from build123d import *
from build123d.topology import SkipClean

# Parameters (mm, degrees)
EXTRUDE_1_DEPTH        = 4
EXTRUDE_3_DEPTH        = 6
CHAMFER_1_SIZE         = 3
SKETCH_5_R             = 0.85
CUT_EXTRUDE_1_DEPTH    = 4
PATTERN_LINEAR_1_COUNT = 4
PATTERN_LINEAR_1_PITCH = 8
CUT_EXTRUDE_2_DEPTH    = 2.5
CUT_EXTRUDE_3_REACH    = 41.439
SKETCH_7_R             = 1.35
SKETCH_8_R             = 6
EXTRUDE_4_DEPTH        = 1.5
FILLET_1_R             = 0.5
SKETCH_9_R             = 5
CUT_EXTRUDE_4_DEPTH    = 3.6
SKETCH_10_R            = 3.55
CUT_EXTRUDE_5_DEPTH    = 3.6
CUT_EXTRUDE_6_DEPTH    = 0.8
CUT_EXTRUDE_7_DEPTH    = 40.958228189
FILLET_2_R             = 2
CHAMFER_2_SIZE         = 1
EXTRUDE_5_DEPTH        = 10


with BuildPart() as part:
    # ｽｹｯﾁ1 → ﾎﾞｽ - 押し出し1 (new body)
    with BuildSketch(Plane(origin=(0, 0, 0), x_dir=(1, 0, 0), z_dir=(0, 1, 0))):
        with BuildLine():
            Line((-7.9, 0), (-7.9, -38))
            Line((-7.9, -38), (7.9, -38))
            Line((7.9, -38), (7.9, 0))
            ThreePointArc((7.9, 0), (0, 7.9), (-7.9, 0))
        make_face()
    extrude(amount=EXTRUDE_1_DEPTH)

    # ｽｹｯﾁ4 → ﾎﾞｽ - 押し出し3 (add)
    with BuildSketch(Plane.XY.offset(38)):
        Polygon((-7, -5.5), (-4.5, -5.5), (-3, -2), (3, -2), (4.5, -5.5), (7, -5.5), (7.9, -2), (7.9, 0), (-7.9, 0), (-7.9, -2), align=None)
    extrude(amount=-EXTRUDE_3_DEPTH)

    # 面取り1
    chamfer_1_edges = [part.edges().sort_by_distance(p)[0] for p in [
        (0, 4, 38),
    ]]
    chamfer(chamfer_1_edges, length=CHAMFER_1_SIZE)

    # ｽｹｯﾁ5 → ｶｯﾄ - 押し出し1 (cut)
    with BuildSketch(Plane(origin=(0, 4, 0), x_dir=(1, 0, 0), z_dir=(0, 1, 0))):
        with Locations(Location((-4, -31, 0), (0, 0, 270))):
            Circle(SKETCH_5_R)
        with Locations(Location((4, -31, 0), (0, 0, 270))):
            Circle(SKETCH_5_R)
    cut_extrude_1 = extrude(amount=-CUT_EXTRUDE_1_DEPTH, mode=Mode.SUBTRACT)

    # 直線ﾊﾟﾀｰﾝ1: ｶｯﾄ - 押し出し1 ×4
    with Locations(*[(0, 0, -i * PATTERN_LINEAR_1_PITCH) for i in range(1, PATTERN_LINEAR_1_COUNT)]):
        add(cut_extrude_1, mode=Mode.SUBTRACT)

    # ｽｹｯﾁ6 → ｶｯﾄ - 押し出し2 (cut)
    with BuildSketch(Plane(origin=(0, 4, 0), x_dir=(1, 0, 0), z_dir=(0, 1, 0))):
        with BuildLine():
            Line((-3, -35), (-3, -39))
            Line((-3, -39), (3, -39))
            Line((3, -39), (3, -35))
            ThreePointArc((3, -35), (0, -32), (-3, -35))
        make_face()
    extrude(amount=-CUT_EXTRUDE_2_DEPTH, mode=Mode.SUBTRACT)

    # ｽｹｯﾁ7 → ｶｯﾄ - 押し出し3 (cut, up to next)
    with BuildSketch(Plane(origin=(0, 1.5, 0), x_dir=(1, 0, 0), z_dir=(0, 1, 0)), mode=Mode.PRIVATE) as cut_extrude_3_sk1:
        with Locations(Location((0, -35, 0), (0, 0, 270))):
            Circle(SKETCH_7_R)
    cut_extrude_3_tool1 = extrude(cut_extrude_3_sk1.sketch, amount=-CUT_EXTRUDE_3_REACH, mode=Mode.PRIVATE) & part.part
    add(cut_extrude_3_tool1.solids().sort_by_distance((0, 1.5, 35))[0], mode=Mode.SUBTRACT)

    # ｽｹｯﾁ8 → ﾎﾞｽ - 押し出し4 (add)
    with BuildSketch(Plane.XZ):
        with Locations(Location((0, 0, 0), (0, 0, 90))):
            Circle(SKETCH_8_R)
    extrude(amount=EXTRUDE_4_DEPTH)

    # ﾌｨﾚｯﾄ1
    fillet_1_edges = [part.edges().sort_by_distance(p)[0] for p in [
        (0, 0, -6),
    ]]
    fillet(fillet_1_edges, radius=FILLET_1_R)

    # ｽｹｯﾁ9 → ｶｯﾄ - 押し出し4 (cut)
    with BuildSketch(Plane(origin=(0, 4, 0), x_dir=(1, 0, 0), z_dir=(0, 1, 0))):
        with Locations(Location((0, 0, 0), (0, 0, 270))):
            Circle(SKETCH_9_R)
    extrude(amount=-CUT_EXTRUDE_4_DEPTH, mode=Mode.SUBTRACT)

    # ｽｹｯﾁ10 → ｶｯﾄ - 押し出し5 (cut)
    with BuildSketch(Plane(origin=(0, 0.4, 0), x_dir=(1, 0, 0), z_dir=(0, 1, 0))):
        with Locations(Location((0, 0, 0), (0, 0, 270))):
            Circle(SKETCH_10_R)
    extrude(amount=-CUT_EXTRUDE_5_DEPTH, mode=Mode.SUBTRACT)

    # ｽｹｯﾁ11 → ｶｯﾄ - 押し出し6 (cut, symmetric)
    with BuildSketch(Plane.XY.offset(35)):
        Polygon((3, -2), (4.5, -5.5), (5.1, -5.5), (3.6, -2), align=None)
        Polygon((7.9, -2), (7, -5.5), (6.4, -5.5), (7.3, -2), align=None)
    cut_extrude_6 = extrude(amount=CUT_EXTRUDE_6_DEPTH, both=True, mode=Mode.SUBTRACT)

    # ﾐﾗｰ1: ｶｯﾄ - 押し出し6 across plane
    add(cut_extrude_6.mirror(Plane(origin=(0, 0, 0), x_dir=(0, 0, 1), z_dir=(1, 0, 0))), mode=Mode.SUBTRACT)

    # ｽｹｯﾁ12 → ｶｯﾄ - 押し出し7 (cut, through all)
    with SkipClean():  # the faces are left unmerged after this step: merging them gives an invalid solid
        with BuildSketch(Plane(origin=(0, 4, 0), x_dir=(1, 0, 0), z_dir=(0, 1, 0))):
            with BuildLine():
                Line((-7.9, 0), (-7.9, -30))
                Line((-7.9, -30), (-6.9, -27))
                Line((-6.9, -27), (-6.9, -3.847076812))
                ThreePointArc((-6.9, -3.847076812), (-7.645913941, -1.987460691), (-7.9, 0))
            make_face()
        cut_extrude_7 = extrude(amount=-CUT_EXTRUDE_7_DEPTH, mode=Mode.SUBTRACT)

    # ﾐﾗｰ2: ｶｯﾄ - 押し出し7 across plane
    with SkipClean():  # the faces are left unmerged after this step: merging them gives an invalid solid
        add(cut_extrude_7.mirror(Plane(origin=(0, 0, 0), x_dir=(0, 0, 1), z_dir=(1, 0, 0))), mode=Mode.SUBTRACT)

    # ﾌｨﾚｯﾄ2
    fillet_2_edges = [part.edges().sort_by_distance(p)[0] for p in [
        (-6.9, 2, 3.847076812),
        (-6.9, 2, 27),
        (-7.9, 2, 30),
        (6.9, 2, 3.847076812),
        (7.9, 2, 30),
        (6.9, 2, 27),
    ]]
    fillet(fillet_2_edges, radius=FILLET_2_R)

    # 面取り2
    # the kernel refuses this chamfer: 1 mm, written as the material it adds along each edge
    with BuildSketch(Plane(origin=(7.9, 0, 32), x_dir=(0, 0.02749587661058639, -0.9996219169112968), z_dir=(-1, 0, 0))) as chamfer_2_piece_1_section:
        Polygon((CHAMFER_2_SIZE * 0.999621916911, CHAMFER_2_SIZE * 0.0274958766106), (-CHAMFER_2_SIZE * 0.0274958766106, CHAMFER_2_SIZE * 0.999621916911), (0, 0), align=None)
    chamfer_2_piece_1 = extrude(amount=15.8, mode=Mode.PRIVATE)
    chamfer_2_piece_1 = chamfer_2_piece_1 - Plane(origin=(-4, -0.34097177, 31), x_dir=(0, 0, 1), z_dir=(0, 1, 0)) * Cylinder(0.85, 36, mode=Mode.PRIVATE)
    chamfer_2_piece_1 = chamfer_2_piece_1 - Plane(origin=(4, -0.34097177, 31), x_dir=(0, 0, 1), z_dir=(0, 1, 0)) * Cylinder(0.85, 36, mode=Mode.PRIVATE)
    add(chamfer_2_piece_1)
    # the kernel refuses this chamfer: 1 mm, written as the material it takes off along each edge
    with BuildSketch(Plane(origin=(-7.9, 4, 30.32455532), x_dir=(-0.027495876610586487, -0.9996219169112968, 0), z_dir=(0, 0, 1)), Plane(origin=(7.9, 4, 37.571682988), x_dir=(0.027495876610586487, -0.9996219169112968, 0), z_dir=(0, 0, -1))) as chamfer_2_2_piece_1:
        Polygon((CHAMFER_2_SIZE * 0.999621916911, CHAMFER_2_SIZE * 0.0274958766106), (-CHAMFER_2_SIZE * 0.0274958766106, CHAMFER_2_SIZE * 0.999621916911), (0, 0), align=None)
    extrude(amount=7.247127668, mode=Mode.SUBTRACT)
    with BuildSketch(Plane(origin=(0, 4, 0), x_dir=(1, 0, 0), z_dir=(0, 0, 1))) as chamfer_2_2_piece_2:
        Polygon((7.9, -CHAMFER_2_SIZE), (7.9 - CHAMFER_2_SIZE, 0), (7.9, 0), align=None)
    revolve(axis=Axis((0, 4, 0), (0, 1, 0)), revolution_arc=180, mode=Mode.SUBTRACT)
    with BuildSketch(Plane(origin=(-5.9, 4, 30.32455532), x_dir=(-1, 0, 0), z_dir=(0, 0, 1))) as chamfer_2_2_piece_3:
        Polygon((2, CHAMFER_2_SIZE), (2 - CHAMFER_2_SIZE, 0), (2, 0), align=None)
    revolve(axis=Axis((-5.9, 4, 30.32455532), (0, -1, 0)), revolution_arc=18.434948823, mode=Mode.SUBTRACT)
    with BuildSketch(Plane(origin=(-7.797366596, 4, 29.692099788), x_dir=(-0.02608487890572092, -0.9996219169112968, -0.008694959635240314), z_dir=(0.3162277660168382, 0, -0.9486832980505138))) as chamfer_2_2_piece_4:
        Polygon((CHAMFER_2_SIZE * 0.999621916911, -CHAMFER_2_SIZE * 0.0274958766106), (-CHAMFER_2_SIZE * 0.0274958766106, -CHAMFER_2_SIZE * 0.999621916911), (0, 0), align=None)
    extrude(amount=2.513167019, mode=Mode.SUBTRACT)
    with BuildSketch(Plane(origin=(-8.9, 4, 26.67544468), x_dir=(0.9486832980505135, 0, 0.3162277660168389), z_dir=(-0.3162277660168389, 0, 0.9486832980505135))) as chamfer_2_2_piece_5:
        Polygon((2, -CHAMFER_2_SIZE), (2 + CHAMFER_2_SIZE, 0), (2, 0), align=None)
    revolve(axis=Axis((-8.9, 4, 26.67544468), (0, 1, 0)), revolution_arc=18.434948823, mode=Mode.SUBTRACT)
    with BuildSketch(Plane(origin=(-6.9, 4, 26.67544468), x_dir=(-0.027495876610586487, -0.9996219169112968, 0), z_dir=(0, 0, -1))) as chamfer_2_2_piece_6:
        Polygon((CHAMFER_2_SIZE * 0.999621916911, -CHAMFER_2_SIZE * 0.0274958766106), (-CHAMFER_2_SIZE * 0.0274958766106, -CHAMFER_2_SIZE * 0.999621916911), (0, 0), align=None)
    extrude(amount=22.339548002, mode=Mode.SUBTRACT)
    with BuildSketch(Plane(origin=(-8.9, 4, 4.335896678), x_dir=(1, 0, 0), z_dir=(0, 0, 1))) as chamfer_2_2_piece_7:
        Polygon((2, -CHAMFER_2_SIZE), (2 + CHAMFER_2_SIZE, 0), (2, 0), align=None)
    revolve(axis=Axis((-8.9, 4, 4.335896678), (0, 1, 0)), revolution_arc=25.974390018, mode=Mode.SUBTRACT)
    with BuildSketch(Plane(origin=(8.9, 4, 4.335896678), x_dir=(-0.8989898989898989, 0, -0.43796936138745074), z_dir=(0.43796936138745074, 0, -0.8989898989898989))) as chamfer_2_2_piece_8:
        Polygon((2, -CHAMFER_2_SIZE), (2 + CHAMFER_2_SIZE, 0), (2, 0), align=None)
    revolve(axis=Axis((8.9, 4, 4.335896678), (0, 1, 0)), revolution_arc=25.974390018, mode=Mode.SUBTRACT)
    with BuildSketch(Plane(origin=(6.9, 4, 26.67544468), x_dir=(0.027495876610586487, -0.9996219169112968, 0), z_dir=(0, 0, -1))) as chamfer_2_2_piece_9:
        Polygon((CHAMFER_2_SIZE * 0.999621916911, CHAMFER_2_SIZE * 0.0274958766106), (-CHAMFER_2_SIZE * 0.0274958766106, CHAMFER_2_SIZE * 0.999621916911), (0, 0), align=None)
    extrude(amount=22.339548002, mode=Mode.SUBTRACT)
    with BuildSketch(Plane(origin=(8.9, 4, 26.67544468), x_dir=(-1, 0, 0), z_dir=(0, 0, -1))) as chamfer_2_2_piece_10:
        Polygon((2, -CHAMFER_2_SIZE), (2 + CHAMFER_2_SIZE, 0), (2, 0), align=None)
    revolve(axis=Axis((8.9, 4, 26.67544468), (0, 1, 0)), revolution_arc=18.434948823, mode=Mode.SUBTRACT)
    with BuildSketch(Plane(origin=(7.797366596, 4, 29.692099788), x_dir=(0.02608487890572092, -0.9996219169112968, -0.008694959635240314), z_dir=(-0.3162277660168382, 0, -0.9486832980505138))) as chamfer_2_2_piece_11:
        Polygon((CHAMFER_2_SIZE * 0.999621916911, CHAMFER_2_SIZE * 0.0274958766106), (-CHAMFER_2_SIZE * 0.0274958766106, CHAMFER_2_SIZE * 0.999621916911), (0, 0), align=None)
    extrude(amount=2.513167019, mode=Mode.SUBTRACT)
    with BuildSketch(Plane(origin=(5.9, 4, 30.32455532), x_dir=(0.9486832980505135, 0, -0.3162277660168389), z_dir=(-0.3162277660168389, 0, -0.9486832980505135))) as chamfer_2_2_piece_12:
        Polygon((2, CHAMFER_2_SIZE), (2 - CHAMFER_2_SIZE, 0), (2, 0), align=None)
    revolve(axis=Axis((5.9, 4, 30.32455532), (0, -1, 0)), revolution_arc=18.434948823, mode=Mode.SUBTRACT)
    with BuildSketch(Plane(origin=(0, 4, 0), x_dir=(0.8989898989898987, 0, 0.43796936138745124), z_dir=(-0.43796936138745124, 0, 0.8989898989898987))) as chamfer_2_2_piece_13:
        Polygon((7.9, -CHAMFER_2_SIZE), (7.9 - CHAMFER_2_SIZE, 0), (7.9, 0), align=None)
    revolve(axis=Axis((0, 4, 0), (0, 1, 0)), revolution_arc=25.974390018, mode=Mode.SUBTRACT)
    with BuildSketch(Plane(origin=(0, 4, 0), x_dir=(-0.8989898989898987, 0, 0.43796936138745124), z_dir=(0.43796936138745124, 0, 0.8989898989898987))) as chamfer_2_2_piece_14:
        Polygon((7.9, CHAMFER_2_SIZE), (7.9 - CHAMFER_2_SIZE, 0), (7.9, 0), align=None)
    revolve(axis=Axis((0, 4, 0), (0, -1, 0)), revolution_arc=25.974390018, mode=Mode.SUBTRACT)

    # Split Bodies 1
    split(bisect_by=Plane.XY.offset(8), keep=Keep.TOP)

    # ｽｹｯﾁ14 → ﾎﾞｽ - 押し出し5 (add)
    with BuildSketch(Plane(origin=(0, 0, 8), x_dir=(-1, 0, 0), z_dir=(0, 0, -1))):
        Polygon((6.9, 0), (-6.9, 0), (-6.9, 3), (-5.9, 4), (5.9, 4), (6.9, 3), align=None)
    extrude(amount=EXTRUDE_5_DEPTH)

    # ﾐﾗｰ3: part across plane


with BuildPart() as part_1:
    add(part.part)
    add(part.part.mirror(Plane(origin=(0, 0, -2), x_dir=(1, 0, 0), z_dir=(0, 0, -1))))


solid = part_1.part
Input: part model. Units: mm. Frame: model coordinates. A direction names the side the tool comes from. Coordinates: 2 decimals unless noted, no trailing zeros. Loops run counter-clockwise (first coordinate to the right, second up) from the corner with the lowest first, then second, coordinate; pieces in that order, holes last. Notation, with made-up numbers: (87.25, 9.25) - (120.25, 9.25) arc R20 cw to (120.25, 41.25) - close; hole circle Ø6 at (-23.5, -0.75). An arc over 180 degrees is marked (long way). Answer in a Markdown table with one row per item. Add a question column.
Item 1: Mould query, pull axis X, two halves, no side actions, for faces 4 (the flat face through (7.9, 0, -38)), 5 (the flat face through (-6.844, -3.774, 35.011)), 6 (the flat face through (-3, 2, -40)). Classes: released by +X, released by -X, zero draft, split by the parting line, or undercut.
Item 2: Section query A-A on z = -19. Return the cut outline in (x, y).
Item 3: Contact query for flat-ended pins moving along their axis: P1, Ø2, axis at x = 5.5, z = 12.5, coming from the -Y side; P2, Ø4, axis at y = 1, z = -17, coming from the -X side. Output: stop coordinate, or through.
Item 4: Line query: line 1 along X through (y, z) = (0.7, -35); line 2 along X through (y, z) = (1.9, -19); line 3 along Z through (x, y) = (-5.5, -2). Output: solid intervals per line, ascending. Write a range as [from, to].
Item 5: Access query for faces 1 (the flat face through (-6.94, 3.49, -32.67)), 2 (the flat face through (-4, -3.7, -38.2)), 3 (the flat face through (-7, -4, -38.2)). Directions: +Z, -Z, +X, -X, +Y, -Y. A direction counts if a zero-diameter tool reaches every point of the face in a straight line with its end or side. Return the directions, or none.
Item 6: Section query C-C on z = 6.5. Return the cut outline in (x, y).
Item 7: Section query B-B on y = -3.75. State how many separate pieces and enclosed holes the cut face has, then the cut area to 3 significant figures.
Recorded:
| question | item | result |
|---|---|---|
| 1 | face 4 | released by +X |
| 1 | face 5 | released by -X |
| 1 | face 6 | undercut |
| 2 | outline | (-6.9, 0) - (-4.85, 0) - (-4.85, 4) - (-5.9, 4) - (-6.9, 3) - close; (-3.15, 0) - (3.15, 0) - (3.15, 4) - (-3.15, 4) - close; (4.85, 0) - (6.9, 0) - (6.9, 3) - (5.9, 4) - (4.85, 4) - close |
| 3 | P1 | y = 0 |
| 3 | P2 | x = -6.9 |
| 4 | line 1 | [-7.9, -4.85], [-3.15, 3.15], [4.85, 7.9] |
| 4 | line 2 | [-6.9, -4.85], [-3.15, 3.15], [4.85, 6.9] |
| 4 | line 3 | [-42, -36], [32, 38] |
| 5 | face 1 | -X, +Y |
| 5 | face 2 | -Y |
| 5 | face 3 | -X, -Y |
| 6 | outline | (-6.9, 0) - (6.9, 0) - (6.9, 3) - (5.9, 4) - (-5.9, 4) - (-6.9, 3) - close |
| 7 | separate pieces | 4 |
| 7 | enclosed holes | 0 |
| 7 | area | 81.1 mm^2 |
